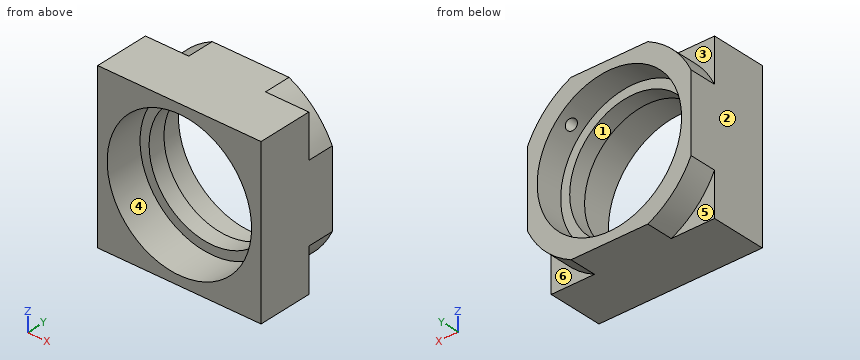
from build123d import *

# Parameters (mm, degrees)
F0_W     = 90.5
F0_H     = 90.5
F1_DEPTH = 45.5
F2_R     = 40
F3_DEPTH = 15
F4_R     = 35
F5_DEPTH = 25
F6_R     = 40
F7_DEPTH = 21
F8_R     = 72.40088581
F8_R_2   = 50
F9_DEPTH = 15


with BuildPart() as f1:
    # F0 (on Front) → F1 (new body)
    with BuildSketch(Plane.XZ):
        Rectangle(F0_W, F0_H)
    extrude(amount=F1_DEPTH)

    # F2 (on face) → F3 (cut)
    with BuildSketch(Plane(origin=(0, 0, 0), x_dir=(-1, 0, 0), z_dir=(0, 1, 0))):
        Circle(F2_R)
    extrude(amount=-F3_DEPTH, mode=Mode.SUBTRACT)

    # F4 (on face) → F5 (cut)
    with BuildSketch(Plane(origin=(0, -15, 0), x_dir=(-1, 0, 0), z_dir=(0, 1, 0))):
        Circle(F4_R)
    extrude(amount=-F5_DEPTH, mode=Mode.SUBTRACT)

    # F6 (on face) → F7 (cut)
    with BuildSketch(Plane.XZ.offset(45.5)):
        Circle(F6_R)
    extrude(amount=-F7_DEPTH, mode=Mode.SUBTRACT)

    # F8 (on face) → F9 (cut)
    with BuildSketch(Plane(origin=(0, 0, 0), x_dir=(-1, 0, 0), z_dir=(0, 1, 0))):
        Circle(F8_R)
        Circle(F8_R_2, mode=Mode.SUBTRACT)
    extrude(amount=-F9_DEPTH, mode=Mode.SUBTRACT)

    # F11 (on offset) → F12 (revolve, cut)
    with BuildSketch(Plane(origin=(0, -8, 0), x_dir=(-1, 0, 0), z_dir=(0, 1, 0))):
        Polygon((-45.1513193548, 45.8626225591), (0, 0), (2.1378338561, 2.1046772683), (-43.0134854987, 47.9672998274), align=None)
    revolve(axis=Axis((22.5756596774, -8, 22.9313112795), (0.7015590894, 0, 0.7126112854)), mode=Mode.SUBTRACT)


solid = f1.part
Can you work these out from the model? Positions are in its coordinate system, mm. Face numbers are marked on the shaded views. A direction names the side the tool comes from. Give positions to 0.01 mm unless a question says otherwise; leave off trailing zeros. Loops run counter-clockwise (first coordinate to the right, second up) from the corner with the lowest first, then second, coordinate; pieces in that order, holes last. Notation, with made-up numbers: (77.5, -9) -> (125.5, -9) arc R20 ccw to (125.5, 9) -> close; hole circle Ø3 at (-26.5, 23). An arc over 180 degrees is marked (long way). Write item = value, one per line.
1) Will this pin go through, and if not, where does the flat tip stop? pin 1 (5 mm diameter, centred on x = 24.5, z = 19.5, fed in from +Y).
Check result:
pin_1 = through
2) I need wall thicknesses on L1, parallel to Z at x = 1, y = -8.5; L2, parallel to Z at x = 0, y = -38; L3, parallel to X at y = -34, z = 13. Which ranges of each line are inside material? Lowest first, please. Write a range as from..to.
Check result:
L1 = -45.25..-39.99, 39.99..45.25
L2 = -45.25..-40, 40..45.25
L3 = -45.25..-37.83, 37.83..45.25
3) Suppose I cut it at A-A on x = 0. Write out the boundary of the cut face in (y, z), then the cut area to 3 significant figures.
Check result:
outline = (-45.5, -45.25) -> (0, -45.25) -> (0, -40) -> (-15, -40) -> (-15, -35) -> (-24.5, -35) -> (-24.5, -40) -> (-45.5, -40) -> close; (-45.5, 40) -> (-24.5, 40) -> (-24.5, 35) -> (-15, 35) -> (-15, 40) -> (0, 40) -> (0, 45.25) -> (-45.5, 45.25) -> close
area = 573 mm2
4) Suppose I cut it at C-C on y = -30.5. Write out the boundary of the cut face in (x, z), then the cut area to 3 significant figures.
Check result:
outline = (-45.25, -45.25) -> (45.25, -45.25) -> (45.25, 45.25) -> (-45.25, 45.25) -> close; hole circle Ø80 at (0, 0)
area = 3,160 mm2
5) Suppose I cut it at B-B on z = 0. Write out the boundary of the cut face in (x, y).
Check result:
outline = (-45.25, -45.5) -> (-40, -45.5) -> (-40, -24.5) -> (-35, -24.5) -> (-35, -15) -> (-40, -15) -> (-40, 0) -> (-45.25, 0) -> close; (35, -24.5) -> (40, -24.5) -> (40, -45.5) -> (45.25, -45.5) -> (45.25, 0) -> (40, 0) -> (40, -15) -> (35, -15) -> close
6) Suppose I cut it at D-D on x = -37.5. Write out the boundary of the cut face in (y, z).
Check result:
outline = (-45.5, -45.25) -> (-15, -45.25) -> (-15, -33.07) -> (0, -33.07) -> (0, -13.92) -> (-15, -13.92) -> (-15, 13.92) -> (0, 13.92) -> (0, 33.07) -> (-15, 33.07) -> (-15, 45.25) -> (-45.5, 45.25) -> (-45.5, 13.92) -> (-24.5, 13.92) -> (-24.5, -13.92) -> (-45.5, -13.92) -> close
7) Thinking about a two-plate mould opening in X: for the marked faces 1, 2 and 3, which applies, released by +X, released by -X, zero draft, split by the parting line, or undercut?
Check result:
face_1 = undercut
face_2 = released by -X
face_3 = zero draft
8) For the marked faces 4, 5 and 6, which set-ups out of +Z, -Z, +X, -X, +Y, -Y let a thin tool reach every point of the face, with its end or its side?
Check result:
face_4 = -Y
face_5 = -Z, -X, +Y
face_6 = -Z, +X, +Y
